from build123d import *

# Parameters (mm, degrees)
SKETCH1_W           = 28.25
SKETCH1_H           = 58
BOSS_EXTRUDE1_DEPTH = 5.9
CUT_EXTRUDE1_REACH  = 7.9
SKETCH2_R           = 2.35
SKETCH2_W           = 20
SKETCH2_H           = 40.5
SKETCH3_W           = 5.9
SKETCH3_H           = 10
BOSS_EXTRUDE2_DEPTH = 5.9
CUT_EXTRUDE2_REACH  = 7.9
SKETCH4_R           = 2.05
CUT_EXTRUDE3_DEPTH  = 10
SKETCH6_W           = 28.25
SKETCH6_H           = 5.9
BOSS_EXTRUDE3_DEPTH = 1
FILLET1_R           = 10
CUT_EXTRUDE4_REACH  = 7.9
SKETCH7_W           = 21
SKETCH7_H           = 41.5


with BuildPart() as part:
    # Sketch1 → Boss-Extrude1 (new body)
    with BuildSketch(Plane(origin=(0, 0, 0), x_dir=(1, 0, 0), z_dir=(0, 1, 0))):
        with Locations((0, 1)):
            Rectangle(SKETCH1_W, SKETCH1_H)
    extrude(amount=BOSS_EXTRUDE1_DEPTH)

    # Sketch2 → Cut-Extrude1 (cut, up to next)
    with BuildSketch(Plane(origin=(0, 5.9, 0), x_dir=(1, 0, 0), z_dir=(0, 1, 0)), mode=Mode.PRIVATE) as cut_extrude1_sk1:
        with Locations((-4.85, -24.3)):
            Circle(SKETCH2_R)
    cut_extrude1_tool1 = extrude(cut_extrude1_sk1.sketch, amount=-CUT_EXTRUDE1_REACH, mode=Mode.PRIVATE) & part.part
    add(cut_extrude1_tool1.solids().sort_by_distance((-4.85, 5.9, 24.3))[0], mode=Mode.SUBTRACT)
    # Sketch2 → Cut-Extrude1 (cut, up to next)
    with BuildSketch(Plane(origin=(0, 5.9, 0), x_dir=(1, 0, 0), z_dir=(0, 1, 0)), mode=Mode.PRIVATE) as cut_extrude1_sk2:
        with Locations((-4.85, 24.8)):
            Circle(SKETCH2_R)
    cut_extrude1_tool2 = extrude(cut_extrude1_sk2.sketch, amount=-CUT_EXTRUDE1_REACH, mode=Mode.PRIVATE) & part.part
    add(cut_extrude1_tool2.solids().sort_by_distance((-4.85, 5.9, -24.8))[0], mode=Mode.SUBTRACT)
    # Sketch2 → Cut-Extrude1 (cut, up to next)
    with BuildSketch(Plane(origin=(0, 5.9, 0), x_dir=(1, 0, 0), z_dir=(0, 1, 0)), mode=Mode.PRIVATE) as cut_extrude1_sk3:
        with Locations((4.85, 24.8)):
            Circle(SKETCH2_R)
    cut_extrude1_tool3 = extrude(cut_extrude1_sk3.sketch, amount=-CUT_EXTRUDE1_REACH, mode=Mode.PRIVATE) & part.part
    add(cut_extrude1_tool3.solids().sort_by_distance((4.85, 5.9, -24.8))[0], mode=Mode.SUBTRACT)
    # Sketch2 → Cut-Extrude1 (cut, up to next)
    with BuildSketch(Plane(origin=(0, 5.9, 0), x_dir=(1, 0, 0), z_dir=(0, 1, 0)), mode=Mode.PRIVATE) as cut_extrude1_sk4:
        with Locations((4.85, -24.3)):
            Circle(SKETCH2_R)
    cut_extrude1_tool4 = extrude(cut_extrude1_sk4.sketch, amount=-CUT_EXTRUDE1_REACH, mode=Mode.PRIVATE) & part.part
    add(cut_extrude1_tool4.solids().sort_by_distance((4.85, 5.9, 24.3))[0], mode=Mode.SUBTRACT)
    # Sketch2 → Cut-Extrude1 (cut, up to next)
    with BuildSketch(Plane(origin=(0, 5.9, 0), x_dir=(1, 0, 0), z_dir=(0, 1, 0)), mode=Mode.PRIVATE) as cut_extrude1_sk5:
        with Locations((0, 0.25)):
            Rectangle(SKETCH2_W, SKETCH2_H)
    cut_extrude1_tool5 = extrude(cut_extrude1_sk5.sketch, amount=-CUT_EXTRUDE1_REACH, mode=Mode.PRIVATE) & part.part
    add(cut_extrude1_tool5.solids().sort_by_distance((0, 5.9, -0.25))[0], mode=Mode.SUBTRACT)

    # Sketch3 → Boss-Extrude2 (add)
    with BuildSketch(Plane(origin=(0, 5.9, 0), x_dir=(1, 0, 0), z_dir=(0, 1, 0))):
        with Locations((-17.075, 0)):
            Rectangle(SKETCH3_W, SKETCH3_H)
        with Locations((17.075, 0)):
            Rectangle(SKETCH3_W, SKETCH3_H)
    extrude(amount=-BOSS_EXTRUDE2_DEPTH)

    # Sketch4 → Cut-Extrude2 (cut, up to next)
    with BuildSketch(Plane(origin=(0, 5.9, 0), x_dir=(1, 0, 0), z_dir=(0, 1, 0)), mode=Mode.PRIVATE) as cut_extrude2_sk1:
        with Locations((-14.125, -5)):
            Circle(SKETCH4_R)
    cut_extrude2_tool1 = extrude(cut_extrude2_sk1.sketch, amount=-CUT_EXTRUDE2_REACH, mode=Mode.PRIVATE) & part.part
    add(cut_extrude2_tool1.solids().sort_by_distance((-14.125, 5.9, 5))[0], mode=Mode.SUBTRACT)
    # Sketch4 → Cut-Extrude2 (cut, up to next)
    with BuildSketch(Plane(origin=(0, 5.9, 0), x_dir=(1, 0, 0), z_dir=(0, 1, 0)), mode=Mode.PRIVATE) as cut_extrude2_sk2:
        with Locations((14.125, -5)):
            Circle(SKETCH4_R)
    cut_extrude2_tool2 = extrude(cut_extrude2_sk2.sketch, amount=-CUT_EXTRUDE2_REACH, mode=Mode.PRIVATE) & part.part
    add(cut_extrude2_tool2.solids().sort_by_distance((14.125, 5.9, 5))[0], mode=Mode.SUBTRACT)

    # Sketch5 → Cut-Extrude3 (cut)
    with BuildSketch(Plane(origin=(0, 5.9, 0), x_dir=(1, 0, 0), z_dir=(0, 1, 0))):
        Polygon((3.1, -20), (3.6, -20), (3.1, -25.5), (-3.1, -25.5), (-3.6, -20), (-3.1, -20), (0, -20), align=None)
    extrude(amount=-CUT_EXTRUDE3_DEPTH, mode=Mode.SUBTRACT)

    # Sketch6 → Boss-Extrude3 (add)
    with BuildSketch(Plane.XY.offset(28)):
        with Locations((0, 2.95)):
            Rectangle(SKETCH6_W, SKETCH6_H)
    extrude(amount=BOSS_EXTRUDE3_DEPTH)

    # Fillet1
    fillet1_edges = [part.edges().sort_by_distance(p)[0] for p in [
        (-14.125, 2.95, 29),
        (14.125, 2.95, 29),
    ]]
    fillet(fillet1_edges, radius=FILLET1_R)

    # Sketch7 → Cut-Extrude4 (cut, up to next)
    with BuildSketch(Plane(origin=(0, 5.9, 0), x_dir=(1, 0, 0), z_dir=(0, 1, 0)), mode=Mode.PRIVATE) as cut_extrude4_sk1:
        with Locations((0, 0.25)):
            Rectangle(SKETCH7_W, SKETCH7_H)
    cut_extrude4_tool1 = extrude(cut_extrude4_sk1.sketch, amount=-CUT_EXTRUDE4_REACH, mode=Mode.PRIVATE) & part.part
    add(cut_extrude4_tool1.solids().sort_by_distance((0, 5.9, -0.25))[0], mode=Mode.SUBTRACT)


solid = part.part
CAD build for the part. Positions are in the model's coordinates, mm. A direction names the side the tool comes from. Coordinates: 2 decimals unless noted, no trailing zeros. Loops run counter-clockwise (first coordinate to the right, second up) from the corner with the lowest first, then second, coordinate; pieces in that order, holes last. Notation, with made-up numbers: (52.25, 32) - (105.25, 32) arc R19 ccw to (105.25, 64) - close; hole circle Ø2 at (57, 70). An arc over 180 degrees is marked (long way). Write item = value, one per line. Start each with the question number.
Q1. Which spindle directions (+Z, -Z, +X, -X, +Y, -Y) get a long thin tool onto all of the face, cutting with end or side? Do faces 1 (the flat face through (-14.125, 3, 13)), 2 (the flat face through (-14.125, 3, -17)), 3 (the flat face through (18, 3, 5)). Say none if no direction does.
Q2. Cut at A-A, the plane x = -0.5. List the corners of the cut face in (y, z).
Q3. Pull direction Z, two halves, no side cores. Call faces 4 (the cylindrical face through (-5.16, 2.99, -27.13)), 5 (the flat face through (-17, 3, -5)), 6 (the cylindrical face through (11.273, 2.991, 25.993)): pulls with the +Z half, pulls with the -Z half, needs draft (parallel to the pull), parting line crosses it, or undercut.
Q4. Flat gauge pins, fed straight in: pin 1 Ø1.9 at (x, y) = (-17, 3.5) entering from +Z; pin 2 Ø4 at (x, z) = (9.5, 21) entering from -Y; pin 3 Ø4 at (x, z) = (4.85, 24.3) entering from +Y (3 decimals); pin 4 Ø3 at (y, z) = (1.5, 22) entering from +X. Where does each tip first touch, or does it go through?
Q5. Cut at C-C, the plane z = 9.5. List the corners of the cut face in (x, y) (3 decimals).
Q6. Drill centre lines: L1, parallel to X at y = 2.05, z = -24.8 (3 decimals); L2, parallel to Z at x = -1, y = 2.5; L3, parallel to X at y = 4.35, z = -8.5 (3 decimals). Where is each one in solid material? Low to high.
Q7. Cut at D-D, the plane y = 2.3. List the corners of the cut face in (x, z) (3 decimals).
Q8. Cut at B-B, the plane z = -24.8. List the corners of the cut face in (x, y) (3 decimals), then the cut area to 3 significant figures.
Computed:
q1.face_1 = +Z, -X, +Y, -Y
q1.face_2 = -Z, -X, +Y, -Y
q1.face_3 = +Z, +X, +Y, -Y
q2.outline = (0, -30) - (5.9, -30) - (5.9, -21) - (0, -21) - close; (0, 25.5) - (5.9, 25.5) - (5.9, 29) - (0, 29) - close
q3.face_4 = undercut
q3.face_5 = pulls with the -Z half
q3.face_6 = pulls with the +Z half
q4.pin_1 = 5
q4.pin_2 = 0
q4.pin_3 = through
q4.pin_4 = 14.01
q5.outline = (-14.125, 0) - (-10.5, 0) - (-10.5, 5.9) - (-14.125, 5.9) - close; (10.5, 0) - (14.125, 0) - (14.125, 5.9) - (10.5, 5.9) - close
q6.L1 = -14.125 to -7.2, -2.5 to 2.5, 7.2 to 14.125
q6.L2 = -30 to -21, 25.5 to 29
q6.L3 = -14.125 to -10.5, 10.5 to 14.125
q7.outline = (-20.025, -5) - (-14.125, -5) - (-14.125, -30) - (14.125, -30) - (14.125, -5) - (20.025, -5) - (20.025, 5) - (16.175, 5) arc R2.05 cw (long way) to (14.125, 7.05) - (14.125, 19) arc R10 ccw to (4.125, 29) - (-4.125, 29) arc R10 ccw to (-14.125, 19) - (-14.125, 7.05) arc R2.05 cw (long way) to (-16.175, 5) - (-20.025, 5) - close; hole (-10.5, -21) - (10.5, -21) - (10.5, 20.5) - (3.555, 20.5) - (3.375, 22.47) arc R2.35 ccw (long way) to (2.829, 25.5) - (-2.829, 25.5) arc R2.35 ccw (long way) to (-3.375, 22.47) - (-3.555, 20.5) - (-10.5, 20.5) - close; hole circle Ø4.7 at (-4.85, -24.8); hole circle Ø4.7 at (4.85, -24.8)
q8.outline = (-14.125, 0) - (-7.2, 0) - (-7.2, 5.9) - (-14.125, 5.9) - close; (-2.5, 0) - (2.5, 0) - (2.5, 5.9) - (-2.5, 5.9) - close; (7.2, 0) - (14.125, 0) - (14.125, 5.9) - (7.2, 5.9) - close
q8.area = 111 mm²
